from build123d import *

# Parameters (mm, degrees)
SKETCH_1_W          = 15.8
SKETCH_1_H          = 47.8
EXTRUDE_1_DEPTH     = 3.2
SKETCH_2_R          = 2.4
EXTRUDE_2_DEPTH     = 1.7
SKETCH_3_R          = 2.5
CUT_EXTRUDE_2_DEPTH = 1.8


with BuildPart() as part:
    # Эскиз1 → Бобышка-Вытянуть1 (new body)
    with BuildSketch(Plane.XY):
        Rectangle(SKETCH_1_W, SKETCH_1_H)
    extrude(amount=EXTRUDE_1_DEPTH)

    # Эскиз2 → Бобышка-Вытянуть2 (add)
    with BuildSketch(Plane.XY.offset(3.2)):
        with Locations(Location((-4, 20, 0), (0, 0, 180))):
            Circle(SKETCH_2_R)
        with Locations(Location((4, 20, 0), (0, 0, 180))):
            Circle(SKETCH_2_R)
        with Locations(Location((4, 12, 0), (0, 0, 180))):
            Circle(SKETCH_2_R)
        with Locations(Location((4, 4, 0), (0, 0, 180))):
            Circle(SKETCH_2_R)
        with Locations(Location((4, -4, 0), (0, 0, 180))):
            Circle(SKETCH_2_R)
        with Locations(Location((4, -12, 0), (0, 0, 180))):
            Circle(SKETCH_2_R)
        with Locations(Location((4, -20, 0), (0, 0, 180))):
            Circle(SKETCH_2_R)
        with Locations(Location((-4, 12, 0), (0, 0, 180))):
            Circle(SKETCH_2_R)
        with Locations(Location((-4, 4, 0), (0, 0, 180))):
            Circle(SKETCH_2_R)
        with Locations(Location((-4, -4, 0), (0, 0, 180))):
            Circle(SKETCH_2_R)
        with Locations(Location((-4, -12, 0), (0, 0, 180))):
            Circle(SKETCH_2_R)
        with Locations(Location((-4, -20, 0), (0, 0, 180))):
            Circle(SKETCH_2_R)
    extrude(amount=EXTRUDE_2_DEPTH)

    # Эскиз3 → Вырез-Вытянуть2 (cut)
    with BuildSketch(Plane(origin=(0, 0, 0), x_dir=(-1, 0, 0), z_dir=(0, 0, -1))):
        with Locations((-4, 20)):
            Circle(SKETCH_3_R)
        with Locations((4, 20)):
            Circle(SKETCH_3_R)
        with Locations((4, 12)):
            Circle(SKETCH_3_R)
        with Locations((4, 4)):
            Circle(SKETCH_3_R)
        with Locations((4, -4)):
            Circle(SKETCH_3_R)
        with Locations((4, -12)):
            Circle(SKETCH_3_R)
        with Locations((4, -20)):
            Circle(SKETCH_3_R)
        with Locations((-4, 12)):
            Circle(SKETCH_3_R)
        with Locations((-4, 4)):
            Circle(SKETCH_3_R)
        with Locations((-4, -4)):
            Circle(SKETCH_3_R)
        with Locations((-4, -12)):
            Circle(SKETCH_3_R)
        with Locations((-4, -20)):
            Circle(SKETCH_3_R)
    extrude(amount=-CUT_EXTRUDE_2_DEPTH, mode=Mode.SUBTRACT)


solid = part.part
Can you work these out from the model? Positions are in its coordinate system, mm. A direction names the side the tool comes from. Give positions to 0.01 mm unless a question says otherwise; leave off trailing zeros. Loops run counter-clockwise (first coordinate to the right, second up) from the corner with the lowest first, then second, coordinate; pieces in that order, holes last. Notation, with made-up numbers: (-10, -29.5) -> (30, -29.5) arc R13 ccw to (30, -4.5) -> close; hole circle Ø8 at (-23.5, -3.75). An arc over 180 degrees is marked (long way). Return JSON: item names as keys, results as strings.
Q1. I want a section at C-C, the plane y = -11. List the corners of the cut face in (x, z) for me.
Checks:
{"outline": "(-7.9, 0) -> (-6.29, 0) -> (-6.29, 1.8) -> (-1.71, 1.8) -> (-1.71, 0) -> (1.71, 0) -> (1.71, 1.8) -> (6.29, 1.8) -> (6.29, 0) -> (7.9, 0) -> (7.9, 3.2) -> (6.18, 3.2) -> (6.18, 4.9) -> (1.82, 4.9) -> (1.82, 3.2) -> (-1.82, 3.2) -> (-1.82, 4.9) -> (-6.18, 4.9) -> (-6.18, 3.2) -> (-7.9, 3.2) -> close"}
Q2. We'd pull the mould along X, two halves only. Please class faces 4 (the face through (-4, -12, 4.9)), 5 (the face through (4, 20, 1.8)): released by +X, released by -X, zero draft, split by the parting line, or undercut.
Checks:
{"face 4": "zero draft", "face 5": "undercut"}
Q3. For pin 1 Ø5.5 at (x, y) = (4, -20) entering from -Z; pin 2 Ø4 at (x, y) = (4, 4) entering from -Z; pin 3 Ø1 at (y, z) = (-16.5, 4) entering from -X; pin 4 Ø1 at (x, z) = (4, 4.5) entering from -Y, each with a flat end and sliding along its axis, tell me the tip position at first contact or that it passes through.
Checks:
{"pin 1": "stops at z = 0", "pin 2": "stops at z = 1.8", "pin 3": "passes through", "pin 4": "stops at y = -22.4"}
Q4. On a 3-axis mill with a long thin cutter (end or side, diameter ignored), from which of +Z, -Z, +X, -X, +Y, -Y can I reach the whole of each face in a straight line? I mean faces 1 (the face through (4.52, -17.657, 4.038)), 2 (the face through (-6.385, 4.751, 0.887)), 3 (the face through (0, 0, 0)). Say none if no direction works.
Checks:
{"face 1": "+Z", "face 2": "-Z", "face 3": "-Z, +X, -X, +Y, -Y"}
Q5. I need wall thicknesses on probe 1 along Y at (x, z) = (-3, 4.45); probe 2 along X at (y, z) = (-6, 1.2); probe 3 along Y at (x, z) = (-5.75, 4.2). Which ranges of each line are inside material? Lowest first, please.
Checks:
{"probe 1": "y = -22.18 to -17.82, -14.18 to -9.82, -6.18 to -1.82, 1.82 to 6.18, 9.82 to 14.18, 17.82 to 22.18", "probe 2": "x = -7.9 to -5.5, -2.5 to 2.5, 5.5 to 7.9", "probe 3": "y = -21.64 to -18.36, -13.64 to -10.36, -5.64 to -2.36, 2.36 to 5.64, 10.36 to 13.64, 18.36 to 21.64"}
Q6. I want a section at D-D, the plane y = -4. List the corners of the cut face in (x, z) for me.
Checks:
{"outline": "(-7.9, 0) -> (-6.5, 0) -> (-6.5, 1.8) -> (-1.5, 1.8) -> (-1.5, 0) -> (1.5, 0) -> (1.5, 1.8) -> (6.5, 1.8) -> (6.5, 0) -> (7.9, 0) -> (7.9, 3.2) -> (6.4, 3.2) -> (6.4, 4.9) -> (1.6, 4.9) -> (1.6, 3.2) -> (-1.6, 3.2) -> (-1.6, 4.9) -> (-6.4, 4.9) -> (-6.4, 3.2) -> (-7.9, 3.2) -> close"}
Q7. I want a section at A-A, the plane z = 3.75. Count the separate pieces of the cut face and the enclosed holes in it, then the cut area to 3 significant figures.
Checks:
{"separate pieces": "12", "enclosed holes": "0", "area": "217 mm2"}
